```python
from build123d import *

# Parameters (mm, degrees)
SKETCH_R        = 60.95906
PAD_DEPTH       = 12
SKETCH001_R     = 5
POCKET_DEPTH    = 12.001
SKETCH002_R     = 2.5
POCKET005_DEPTH = 357.671689
POCKET004_DEPTH = 357.671689


with BuildPart() as part:
    # Sketch → Pad (new body)
    with BuildSketch(Plane.XY):
        Circle(SKETCH_R)
    extrude(amount=PAD_DEPTH)

    # Sketch001 → Pocket (cut, through all)
    with BuildSketch(Plane(origin=(0, 0, 0), x_dir=(-1, 0, 0), z_dir=(0, 0, -1))):
        Circle(SKETCH001_R)
    extrude(amount=-POCKET_DEPTH, mode=Mode.SUBTRACT)

    # Sketch002 → Pocket005 (cut, through all)
    with BuildSketch(Plane(origin=(0, 0, 0), x_dir=(-1, 0, 0), z_dir=(0, 0, -1))):
        with Locations((12.5, 20.5)):
            Circle(SKETCH002_R)
        with Locations((12.5, -20.5)):
            Circle(SKETCH002_R)
    pocket005 = extrude(amount=-POCKET005_DEPTH, mode=Mode.SUBTRACT)

    # Mirrored001: Pocket005 across Sketch002 V_Axis
    add(pocket005.mirror(Plane(origin=(0, 0, 0), x_dir=(0, 0, -1), z_dir=(-1, 0, 0))), mode=Mode.SUBTRACT)

    # Sketch005 → Pocket004 (cut, through all)
    with BuildSketch(Plane(origin=(0, 0, 0), x_dir=(-1, 0, 0), z_dir=(0, 0, -1))):
        with BuildLine():
            Line((12.5, 10.5), (49.622697, 10.5))
            ThreePointArc((49.622697, 10.5), (56.193721, 13.936925), (57.118715, 21.294587))
            ThreePointArc((57.118706, -21.294612), (60.95906, -1.3e-05), (57.118715, 21.294587))
            ThreePointArc((57.118706, -21.294612), (56.193728, -13.936936), (49.622697, -10.5))
            Line((12.5, -10.5), (49.622697, -10.5))
            Line((12.5, 0), (12.5, -10.5))
            Line((12.5, 10.5), (12.5, 0))
        make_face()
    pocket004 = extrude(amount=-POCKET004_DEPTH, mode=Mode.SUBTRACT)

    # Mirrored: Pocket004 across Sketch005 V_Axis
    add(pocket004.mirror(Plane(origin=(0, 0, 0), x_dir=(0, 0, -1), z_dir=(-1, 0, 0))), mode=Mode.SUBTRACT)


solid = part.part
```
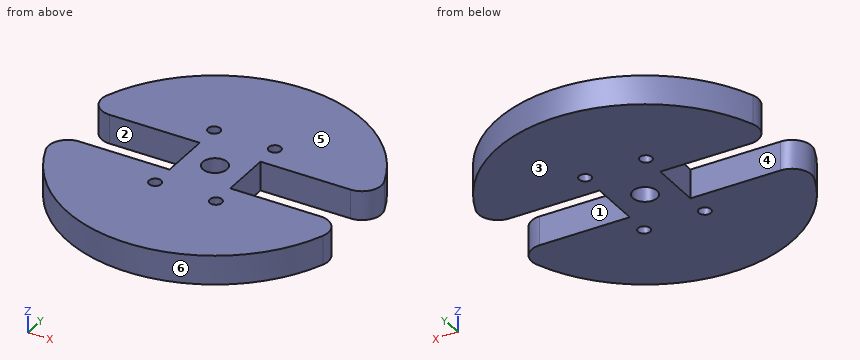
Check sheet for the modelled part. Datum: model origin and axes. Units: mm. Face numbers are marked on the shaded views. A direction names the side the tool comes from. Give positions to 0.01 mm unless a question says otherwise; leave off trailing zeros. Loops run counter-clockwise (first coordinate to the right, second up) from the corner with the lowest first, then second, coordinate; pieces in that order, holes last. Notation, with made-up numbers: (-34.5, 20) - (23.5, 20) arc R7 ccw to (23.5, 29) - close; hole circle Ø5 at (17, 75). An arc over 180 degrees is marked (long way). One line per question, with ' | ' between items. Start each with the question number.
1. Set-up check for the marked faces 1, 2 and 3: record each of +Z, -Z, +X, -X, +Y, -Y from which the full face is reachable in a straight line by a thin tool's end or side.
2. Gauge pin test, flat ends, axial feed: pin 1 Ø3.5 at (x, z) = (-40, 6) entering from +Y; pin 2 Ø3.5 at (x, z) = (32, 3.5) entering from +Y; pin 3 Ø3 at (x, z) = (-43, 6) entering from -Y. Record the tip position at first contact, or that the pin passes through.
3. Cross-section at B-B, the plane x = 0. Enter the section's corners in (y, z).
4. Draft check along Y on the marked faces 4, 5 and 6. Enter one of: released by +Y, released by -Y, zero draft, split by the parting line, or undercut.
5. Material ranges on line 1 along Y through (x, z) = (0, 9.75); line 2 along Y through (x, z) = (14, 7); line 3 along X through (y, z) = (18.5, 1.5), recorded low to high. Write a range as [from, to].
6. Cross-section at C-C, the plane z = 4.5. Enter the section's corners in (x, y).
7. Cross-section at A-A, the plane y = 0. Enter the section's corners in (x, z).
Check result:
1) face 1: +Z, -Z, +X | face 2: +Z, -Z, -X | face 3: -Z, +X, -X, +Y, -Y
2) pin 1: stops at y = 47.47 | pin 2: stops at y = 52.92 | pin 3: stops at y = -44.65
3) outline: (-60.96, 0) - (-5, 0) - (-5, 12) - (-60.96, 12) - close; (5, 0) - (60.96, 0) - (60.96, 12) - (5, 12) - close
4) face 4: undercut | face 5: zero draft | face 6: released by -Y
5) line 1: y = [-60.96, -5], [5, 60.96] | line 2: y = [-59.33, -22.5], [-18.5, -10.5], [10.5, 18.5], [22.5, 59.33] | line 3: x = [-57.62, -14], [-11, 11], [14, 57.62]
6) outline: (-57.12, -21.29) arc R60.96 ccw to (57.12, -21.29) arc R8 ccw to (49.62, -10.5) - (12.5, -10.5) - (12.5, 10.5) - (49.62, 10.5) arc R8 ccw to (57.12, 21.29) arc R60.96 ccw to (-57.12, 21.29) arc R8 ccw to (-49.62, 10.5) - (-12.5, 10.5) - (-12.5, -10.5) - (-49.62, -10.5) arc R8 ccw to start; hole circle Ø5 at (-12.5, -20.5); hole circle Ø5 at (-12.5, 20.5); hole circle Ø10 at (0, 0); hole circle Ø5 at (12.5, -20.5); hole circle Ø5 at (12.5, 20.5)
7) outline: (-12.5, 0) - (-5, 0) - (-5, 12) - (-12.5, 12) - close; (5, 0) - (12.5, 0) - (12.5, 12) - (5, 12) - close
